Geometry check sheet. Reference: the model listing, model coordinates, mm. Face numbers are marked on the shaded views. Round coordinates to 2 decimals unless told otherwise and drop trailing zeros. Order: outer loops, then holes, each group sorted by start corner. A loop starts at its lowest first (then second) coordinate and runs counter-clockwise, first axis right, second up. Notation, with made-up numbers: (77.5, -21) - (113.5, -21) arc R16 ccw to (113.5, 8) - close; hole circle Ø10 at (32.25, 33). An arc over 180 degrees is marked (long way). Use a Markdown table: item, result. Add a question column.
(1) Section check A-A on z = -0.75. Record the boundary of the cut face in (x, y).
(2) Gauge pin test, flat ends, axial feed: P1, Ø1.5, axis at x = 2, z = -4.5, coming from the +Y side; P2, Ø2, axis at x = -0.5, z = -5.5, coming from the -Y side; P3, Ø1, axis at y = 0.5, z = -12, coming from the +X side. Record the tip position at first contact, or that the pin passes through.
(3) Mould release check, pull along Y, two halves, no side actions. Record for the marked faces 1, 2 and 3: released by +Y, released by -Y, zero draft, split by the parting line, or undercut.
(4) Thickness scan on line 1 along Z through (x, y) = (-1.9, -0.75); line 2 along X through (y, z) = (0, -4); line 3 along Y through (x, z) = (0.3, -0.75). Record the ranges inside material, lowest first. Write a range as [from, to].
(5) Section check B-B on z = -4.75. Record the boundary of the cut face in (x, y), then the cut area to 3 significant figures.
```python
from build123d import *

# Parameters (mm, degrees)
CUT_EXTRUDE1_DEPTH = 1.3


with BuildPart() as part:
    # Sketch1 → Revolve1 (revolve)
    with BuildSketch(Plane(origin=(0, 0, 0), x_dir=(0, 0, -1), z_dir=(1, 0, 0))):
        with BuildLine():
            Line((0, 0), (0, 2.45))
            Line((0, 2.45), (0.3, 2.75))
            Line((0.3, 2.75), (2.785, 2.75))
            Line((2.785, 2.75), (3, 2.535))
            Line((3, 2.535), (3, 1.8))
            ThreePointArc((3, 1.8), (3.015193643, 1.74701055), (3.056157637, 1.710123155))
            Line((3.056157637, 1.710123155), (3.466157637, 1.510123155))
            ThreePointArc((3.466157637, 1.510123155), (3.48750205, 1.50256365), (3.51, 1.5))
            Line((3.51, 1.5), (14.75, 1.5))
            Line((14.75, 1.5), (15, 1.25))
            Line((15, 1.25), (15, 0))
            Line((15, 0), (0, 0))
        make_face()
    revolve(axis=Axis((0, 0, 0), (0, 0, -1)))

    # Sketch2 → Cut-Extrude1 (cut)
    with BuildSketch(Plane.XY):
        Polygon((0, 1.443375673), (-1.25, 0.721687836), (-1.25, -0.721687836), (0, -1.443375673), (1.25, -0.721687836), (1.25, 0.721687836), align=None)
    extrude(amount=-CUT_EXTRUDE1_DEPTH, mode=Mode.SUBTRACT)

    # Sketch3 → Cut-Revolve2 (revolve, cut)
    with BuildSketch(Plane(origin=(0, 0, 0), x_dir=(0, 0, -1), z_dir=(1, 0, 0))):
        Polygon((1.3, 0), (1.3, 1.25), (2.021687836, 0), align=None)
    revolve(axis=Axis((0, 0, -1.3), (0, 0, -1)), mode=Mode.SUBTRACT)

    # Sketch4 → Cut-Revolve3 (revolve, cut)
    with BuildSketch(Plane(origin=(0, 0, 0), x_dir=(0, 0, -1), z_dir=(1, 0, 0))):
        Polygon((0, 1.443375673), (0, 1.25), (0.051814855, 1.25), align=None)
    revolve(axis=Axis((0, 0, 0), (0, 0, -1)), mode=Mode.SUBTRACT)


solid = part.part
```
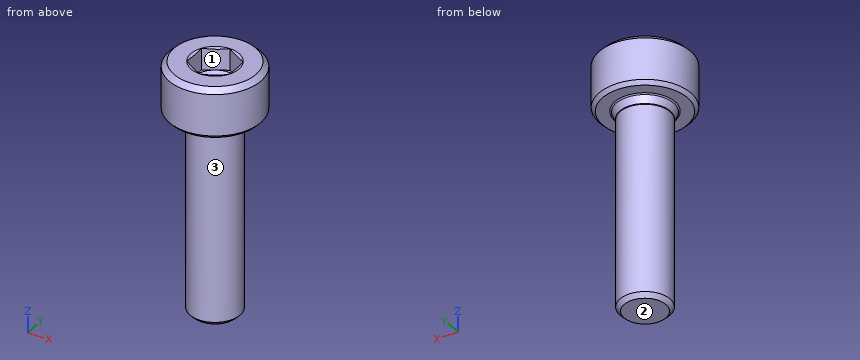
Check sheet entries:
| question | item | result |
|---|---|---|
| 1 | outline | circle Ø5.5 at (0, 0); hole (-1.25, -0.72) - (0, -1.44) - (1.25, -0.72) - (1.25, 0.72) - (0, 1.44) - (-1.25, 0.72) - close |
| 2 | P1 | stops at y = 0.83 |
| 2 | P2 | stops at y = -1.5 |
| 2 | P3 | stops at x = 1.5 |
| 3 | face 1 | undercut |
| 3 | face 2 | zero draft |
| 3 | face 3 | split by the parting line |
| 4 | line 1 | z = [-3, 0] |
| 4 | line 2 | x = [-1.5, 1.5] |
| 4 | line 3 | y = [-2.73, -1.27], [1.27, 2.73] |
| 5 | outline | circle Ø3 at (0, 0) |
| 5 | area | 7.07 mm2 |
